Could you check a few things on this model? Use its own coordinates, in mm. A direction names the side the tool comes from. Give positions to 0.01 mm unless a question says otherwise; leave off trailing zeros. Order: outer loops, then holes, each group sorted by start corner. A loop starts at its lowest first (then second) coordinate and runs counter-clockwise, first axis right, second up. Notation, with made-up numbers: (9.25, 4.5) - (57.25, 4.5) arc R8 cw to (57.25, 17.5) - close; hole circle Ø6 at (-27, 88). An arc over 180 degrees is marked (long way). Put each result on its own line as item: value.
from build123d import *

# Parameters (mm, degrees)
F0_W     = 1910
F0_H     = 40
F1_DEPTH = 100
F2_W     = 100
F2_H     = 40
F3_DEPTH = 450
F4_R     = 99.99999


# Not quite as in the source:
# - a fillet or chamfer is up to 0.001 mm smaller than in the source, because OpenCascade refuses the exact size


with BuildPart() as f1:
    # F0 (on Top) → F1 (new body)
    with BuildSketch(Plane.XY):
        with Locations((10.5278193951, -112.9367578724)):
            Rectangle(F0_W, F0_H)
    extrude(amount=F1_DEPTH)

    # F2 (on face) → F3 (join)
    with BuildSketch(Plane.XY.offset(100)):
        with Locations((915.5278193951, -112.9367578724)):
            Rectangle(F2_W, F2_H)
    extrude(amount=F3_DEPTH)

    # F4 (radius 100 in the source; OpenCascade refuses exactly that, so slightly less here)
    f4_edges = [f1.edges().sort_by_distance(p)[0] for p in [
        (-944.472181, -112.936758, 100),
        (865.527819, -112.936758, 550),
    ]]
    fillet(f4_edges, radius=F4_R)


solid = f1.part
1) If I drill on line 1 (Z direction, x = -277, y = -125.5); line 2 (X direction, y = -126.5, z = 356); line 3 (Z direction, x = 879, y = -108.5), over which ranges is the centre line in solid material (lowest first)? Write a range as [from, to].
Filled in:
line 1: z = [0, 100]
line 2: x = [865.53, 965.53]
line 3: z = [0, 500.13]
2) Which directions (+Z, -Z, +X, -X, +Y, -Y) give clear straight access to the entire face, cutting with the end or side of a thin tool? Please do faces 1 (the flat face through (865.528, -113, 273)), 2 (the flat face through (148, -132.937, 90)).
Filled in:
face 1: +Z, -X, +Y, -Y
face 2: +Z, -Z, +X, -X, -Y
3) Suppose I cut it at B-B, the plane x = -793. List the corners of the cut face in (y, z) for me.
Filled in:
outline: (-132.94, 0) - (-92.94, 0) - (-92.94, 100) - (-132.94, 100) - close
4) Suppose I cut it at C-C, the plane z = 217.5. List the corners of the cut face in (x, y) for me, and give its area (3 significant figures).
Filled in:
outline: (865.53, -132.94) - (965.53, -132.94) - (965.53, -92.94) - (865.53, -92.94) - close
area: 4,000 mm^2
5) I'm going to push flat-ended pins straight in: pin 1 (6 mm diameter, centred on x = -59, y = -126.5, fed in from -Z); pin 2 (12 mm diameter, centred on y = -104.5, z = 265.5, fed in from -X); pin 3 (8 mm diameter, centred on x = 12.5, y = -99.5, fed in from +Z). Where does each tip first touch, or does it pass through?
Filled in:
pin 1: stops at z = 0
pin 2: stops at x = 865.53
pin 3: stops at z = 100
